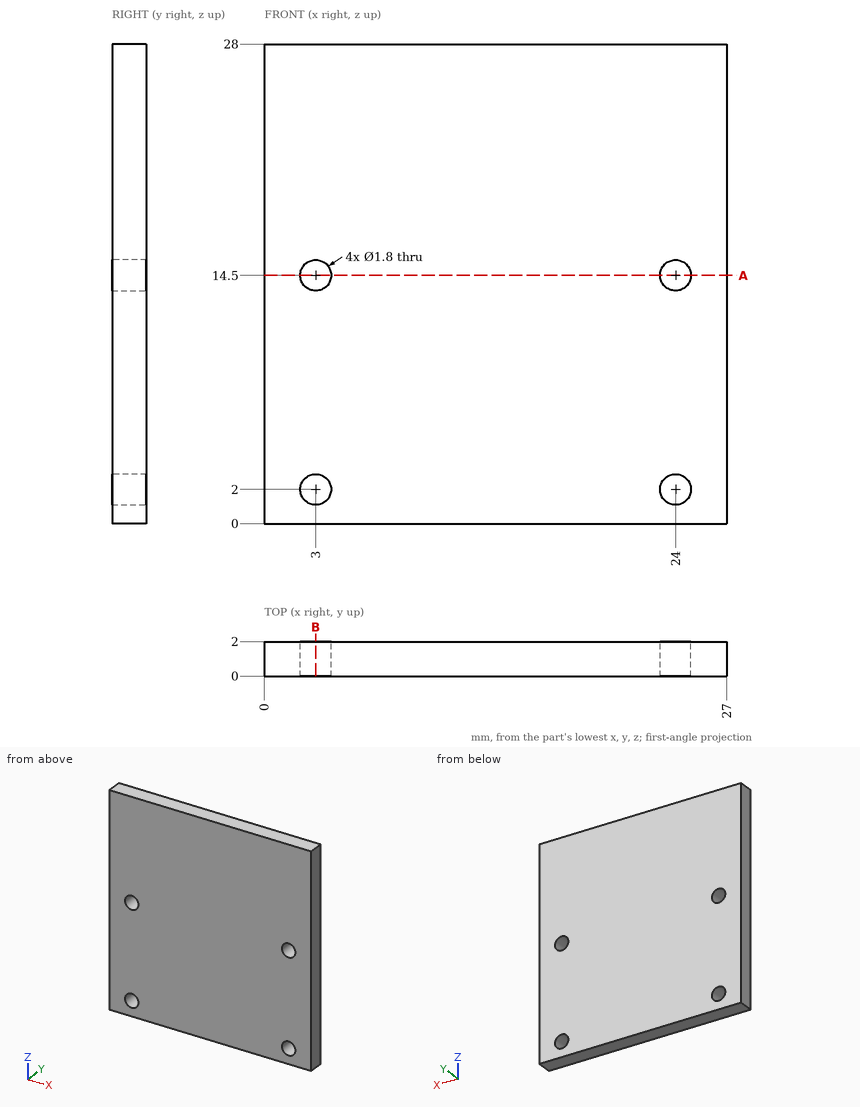
Part print with two shaded views. Sizes in mm from the minimum x, y, z corner. Coordinates: 2 decimals unless noted, no trailing zeros. Write each loop counter-clockwise with the first axis right and the second up, starting at its lowest first coordinate (ties: lowest second). Pieces come first, ordered by that corner, then holes. Notation, with made-up numbers: (2, 65) - (35, 65) arc R14 cw to (35, 77) - close; hole circle Ø5 at (19.5, 24). An arc over 180 degrees is marked (long way). One line per item, written item: value. Start each with the question number.
1. Slice it at B-B (x = 3). Write the cut outline in (y, z), plus the area to 3 significant figures.
2. Flat gauge pins, fed straight in: pin 1 (1.1 mm diameter, centred on x = 3, z = 2, fed in from -Y); pin 2 (4 mm diameter, centred on x = 15, z = 18, fed in from -Y). Where does each tip first touch, or does it go through?
3. Slice it at A-A (z = 14.5). Write the cut outline in (x, y), plus the area to 3 significant figures.
4. Probe line 1 (X direction, y = 1.4, z = 2); line 2 (Z direction, x = 2.5, y = 1.2); line 3 (X direction, y = 0.45, z = 1.5). List the from-to ranges inside material, lowest first. Write a range as from..to.
Answers below:
1. outline: (0, 0) - (2, 0) - (2, 1.1) - (0, 1.1) - close; (0, 2.9) - (2, 2.9) - (2, 13.6) - (0, 13.6) - close; (0, 15.4) - (2, 15.4) - (2, 28) - (0, 28) - close
1. area: 48.8 mm^2
2. pin 1: passes through
2. pin 2: stops at y = 0
3. outline: (0, 0) - (2.1, 0) - (2.1, 2) - (0, 2) - close; (3.9, 0) - (23.1, 0) - (23.1, 2) - (3.9, 2) - close; (24.9, 0) - (27, 0) - (27, 2) - (24.9, 2) - close
3. area: 46.8 mm^2
4. line 1: x = 0..2.1, 3.9..23.1, 24.9..27
4. line 2: z = 0..1.25, 2.75..13.75, 15.25..28
4. line 3: x = 0..2.25, 3.75..23.25, 24.75..27
